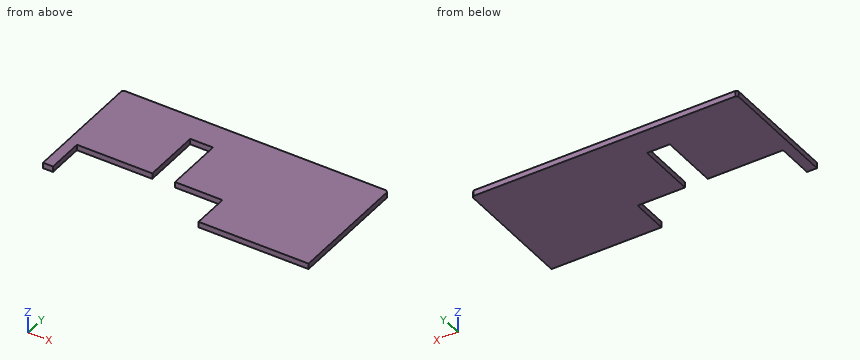
Solid Edge part; units mm, degrees
sketch "Sketch1" plane through (0, 0, 0) normal (0, 0, 1) x (1, 0, 0)
  line L0 (75, 32.5) -> (-65, 32.5)
  line L1 (-65, 32.5) -> (-65, -32.5)
  line L2 (-59.72, -32.5) -> (-65, -32.5)
  line L3 (-59.72, -32.5) -> (-59.72, -13)
  line L4 (-20, -13) -> (-59.72, -13)
  line L5 (-20, -13) -> (-20, 17.97)
  line L6 (-20, 17.97) -> (-8, 17.97)
  line L7 (-8, 17.97) -> (-8, -13)
  line L8 (-8, -13) -> (17, -13)
  line L9 (17, -13) -> (17, -32.5)
  line L10 (17, -32.5) -> (75, -32.5)
  line L11 (75, -32.5) -> (75, 32.5)
extrude "Protrusion1" add sketch "Sketch1" against normal blind 3
chamfer "Chanfro_1" distance 1 angle 45 1 edges at (75, 32.5, -1.5)
chamfer "Chanfro_2" distance 1 angle 45 1 edges at (-65, 32.5, -1.5)
Could you check a few things on this model? Use its own coordinates, in mm. Give positions to 0.01 mm unless a question says otherwise; leave off trailing zeros. Write each loop counter-clockwise with the first axis right and the second up, starting at its lowest first coordinate (ties: lowest second). Pieces come first, ordered by that corner, then holes. Notation, with made-up numbers: (75.5, 15) -> (127.5, 15) arc R28 cw to (127.5, 43) -> close; hole circle Ø4 at (88, -28). An arc over 180 degrees is marked (long way). Write each question's results on one line, items separated by ' | '.
1. I want a section at B-B, the plane z = -1.95. Write out the boundary of the cut face in (x, y).
Check sheet entries:
outline: (-65, -32.5) -> (-59.72, -32.5) -> (-59.72, -13) -> (-20, -13) -> (-20, 17.97) -> (-8, 17.97) -> (-8, -13) -> (17, -13) -> (17, -32.5) -> (75, -32.5) -> (75, 31.5) -> (74, 32.5) -> (-64, 32.5) -> (-65, 31.5) -> close
2. I want a section at A-A, the plane y = -1. Write out the boundary of the cut face in (x, z).
Check sheet entries:
outline: (-65, -3) -> (-20, -3) -> (-20, 0) -> (-65, 0) -> close; (-8, -3) -> (75, -3) -> (75, 0) -> (-8, 0) -> close
3. I need wall thicknesses on L1, parallel to X at y = -2, z = -1.2; L2, parallel to X at y = -13.5, z = -1.75; L3, parallel to Y at x = -14, z = -2.2. Which ranges of each line are inside material? Lowest first, please.
Check sheet entries:
L1: x = -65 to -20, -8 to 75 | L2: x = -65 to -59.72, 17 to 75 | L3: y = 17.97 to 32.5
4. Will these pins go through, and if not, where does the flat tip stop? pin 1 Ø8 at (x, y) = (15.5, 20) entering from +Z; pin 2 Ø1.5 at (x, z) = (-0.5, -1) entering from -Y.
Check sheet entries:
pin 1: stops at z = 0 | pin 2: stops at y = -13
5. I want a section at D-D, the plane x = 10.5. Write out the boundary of the cut face in (y, z), then the cut area to 4 significant figures.
Check sheet entries:
outline: (-13, -3) -> (32.5, -3) -> (32.5, 0) -> (-13, 0) -> close | area: 136.5 mm²
6. I want a section at C-C, the plane x = -13. Write out the boundary of the cut face in (y, z).
Check sheet entries:
outline: (17.97, -3) -> (32.5, -3) -> (32.5, 0) -> (17.97, 0) -> close
